Part model, mm, in its own coordinate system. A direction names the side the tool comes from. Round coordinates to 2 decimals unless told otherwise and drop trailing zeros. Order: outer loops, then holes, each group sorted by start corner. A loop starts at its lowest first (then second) coordinate and runs counter-clockwise, first axis right, second up. Notation, with made-up numbers: (36, 20.5) - (75, 20.5) arc R27 ccw to (75, 55.5) - close; hole circle Ø10 at (54.5, 1). An arc over 180 degrees is marked (long way). Return JSON: item names as keys, results as strings. Group by question number.
Item 1: Two-plate mould, pull along X, no slides. Class faces 3 (the face through (0, 3, 1.993)), 4 (the face through (1.802, 2.958, 5.723)), 5 (the face through (-3, 6, 0)): released by +X, released by -X, zero draft, split by the parting line, or undercut.
Item 2: Saw through at D-D on z = 4. List the corners of the cut face in (x, y), and give its area (3 significant figures).
Item 3: Saw through at B-B on z = 0. List the corners of the cut face in (x, y), and give its area (3 significant figures).
Item 4: Saw through at C-C on y = 4.35. List the corners of the cut face in (x, z), and give its area (3 significant figures).
Item 5: Tool access for faces 1 (the face through (-3, 0, 0)), 2 (the face through (-1.491, 3, 0)): list every direction of +Z, -Z, +X, -X, +Y, -Y with a clear straight run to the whole face (end or side of a thin tool).
Item 6: Drop flat-ended pins along their axis: pin 1 (2 mm diameter, centred on y = 2.5, z = 3, fed in from +X); pin 2 (2 mm diameter, centred on y = 2, z = -4, fed in from +X); pin 3 (1 mm diameter, centred on y = 2.5, z = 2, fed in from +X). Give the stop position or say it passes through.
Item 7: Saw through at A-A on x = 0. List the corners of the cut face in (y, z), and give its area (3 significant figures).
Item 8: Probe probe 1 along X at (y, z) = (3.4, 0); probe 2 along X at (y, z) = (3.95, -1.5); probe 3 along Z at (x, y) = (2.5, 2.7). List the from-to ranges inside material, lowest first.
```python
from build123d import *

# Parameters (mm, degrees)
SKETCH_1_R          = 6
SKETCH_1_R_2        = 2.5
EXTRUDE_4_DEPTH     = 6
SKETCH_2_W          = 2.981877758
SKETCH_2_H          = 3.986343956
CUT_EXTRUDE_1_DEPTH = 10


with BuildPart() as part:
    # 草图1 → 凸台-拉伸4 (new body)
    with BuildSketch(Plane(origin=(0, 0, 0), x_dir=(1, 0, 0), z_dir=(0, 1, 0))):
        with Locations(Location((0, 0, 0), (0, 0, 270))):
            Circle(SKETCH_1_R)
        with Locations(Location((3, 0, 0), (0, 0, 270))):
            Circle(SKETCH_1_R_2, mode=Mode.SUBTRACT)
    extrude(amount=EXTRUDE_4_DEPTH)

    # 草图2 → 切除-拉伸1 (cut)
    with BuildSketch(Plane(origin=(0, 6, 0), x_dir=(1, 0, 0), z_dir=(0, 1, 0))):
        Rectangle(SKETCH_2_W, SKETCH_2_H)
    extrude(amount=-CUT_EXTRUDE_1_DEPTH, mode=Mode.SUBTRACT)


solid = part.part
```
Filled in:
{
 "1": {"face 3": "undercut", "face 4": "split by the parting line", "face 5": "zero draft"},
 "2": {"outline": "(-4.47, 0) - (4.47, 0) - (4.47, 6) - (-4.47, 6) - close", "area": "53.7 mm^2"},
 "3": {"outline": "(-6, 0) - (-1.49, 0) - (-1.49, 6) - (-6, 6) - close; (5.5, 0) - (6, 0) - (6, 6) - (5.5, 6) - close", "area": "30.1 mm^2"},
 "4": {"outline": "circle Ø12 at (0, 0); hole (-1.49, -1.99) - (1.49, -1.99) arc R2.5 ccw (long way) to (1.49, 1.99) - (-1.49, 1.99) - close", "area": "84.3 mm^2"},
 "5": {"face 1": "+Z, -Z, +X, -X, -Y", "face 2": "+Y, -Y"},
 "6": {"pin 1": "stops at x = 5.66", "pin 2": "stops at x = 5.2", "pin 3": "stops at x = 5.81"},
 "7": {"outline": "(0, -6) - (6, -6) - (6, -1.99) - (0, -1.99) - close; (0, 1.99) - (6, 1.99) - (6, 6) - (0, 6) - close", "area": "48.1 mm^2"},
 "8": {"probe 1": "x = -6 to -1.49, 5.5 to 6", "probe 2": "x = -5.81 to -1.49, 5 to 5.81", "probe 3": "z = -5.45 to -2.45, 2.45 to 5.45"}
}
